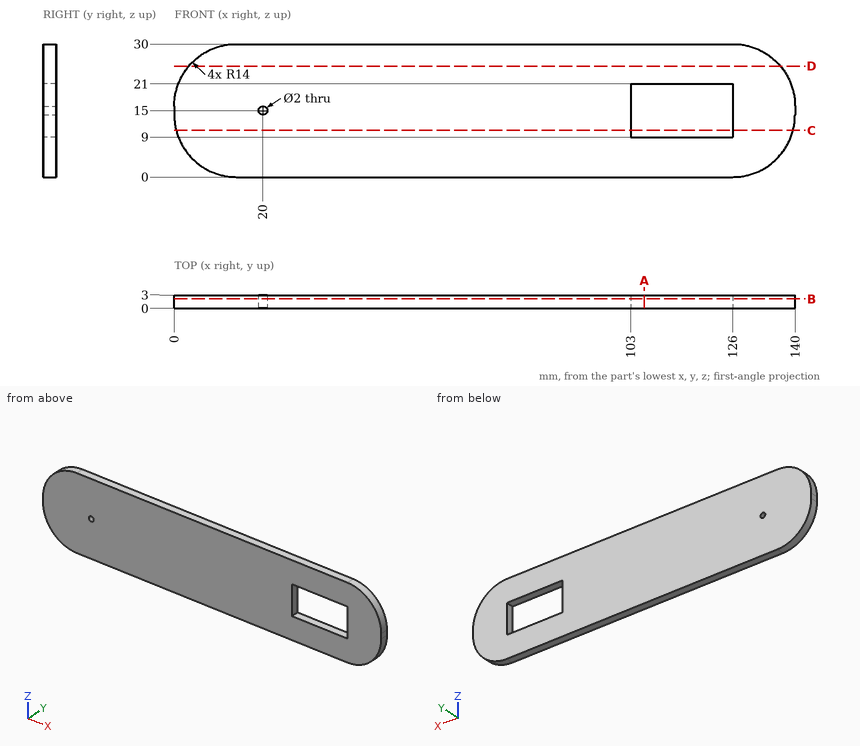
Design review of the part shown in the three views and the two pictorial views. Dimensions are in mm from the part's minimum x, y and z. Coordinates: 2 decimals unless noted, no trailing zeros. Write each loop counter-clockwise with the first axis right and the second up, starting at its lowest first coordinate (ties: lowest second). Pieces come first, ordered by that corner, then holes. Notation, with made-up numbers: (8.25, -18) - (19.25, -18) arc R17 ccw to (19.25, -6) - close; hole circle Ø5 at (-23, 70.5). An arc over 180 degrees is marked (long way). Write item = value, one per line.
(1) Consider section A-A, the plane x = 106. Give the boundary of the cut face in (y, z), then the cut area to 3 significant figures.
Result sheet:
outline = (0, 0) - (3, 0) - (3, 9) - (0, 9) - close; (0, 21) - (3, 21) - (3, 30) - (0, 30) - close
area = 54.0 mm^2
(2) Consider section B-B, the plane y = 2.15. Give the boundary of the cut face in (x, z).
Result sheet:
outline = (0, 14) arc R14 ccw to (14, 0) - (126, 0) arc R14 ccw to (140, 14) - (140, 16) arc R14 ccw to (126, 30) - (14, 30) arc R14 ccw to (0, 16) - close; hole circle Ø2 at (20, 15); hole (103, 9) - (126, 9) - (126, 21) - (103, 21) - close
(3) Consider section C-C, the plane z = 10.5. Give the boundary of the cut face in (x, y), then the cut area to 3 significant figures.
Result sheet:
outline = (0.44, 0) - (103, 0) - (103, 3) - (0.44, 3) - close; (126, 0) - (139.56, 0) - (139.56, 3) - (126, 3) - close
area = 348 mm^2
(4) For line 1 (X direction, y = 0.95, z = 15); line 2 (Z direction, x = 20, y = 2.15); line 3 (X direction, y = 1.45, z = 15.75), list the stretches that pass through material, from the lowest coordinate up. Write a range as [from, to].
Result sheet:
line_1 = [0, 19], [21, 103], [126, 140]
line_2 = [0, 14], [16, 30]
line_3 = [0, 19.34], [20.66, 103], [126, 140]
(5) For P1, Ø1, axis at y = 1.5, z = 9, coming from the +X side, flat-tipped, find the tip position at first contact; note if it passes through.
Result sheet:
P1 = 139.26
(6) Consider section D-D, the plane z = 25. Give the boundary of the cut face in (x, y), then the cut area to 3 significant figures.
Result sheet:
outline = (3.28, 0) - (136.72, 0) - (136.72, 3) - (3.28, 3) - close
area = 400 mm^2
